```python
from build123d import *

# Parameters (mm, degrees)
SKETCH_1_W      = 100
SKETCH_1_H      = 100
EXTRUDE_1_DEPTH = 3
SKETCH_4_W      = 100
SKETCH_4_H      = 100
EXTRUDE_4_DEPTH = 33
FILLET_3_R      = 8
SKETCH_7_R      = 3.25
EXTRUDE_6_DEPTH = 33


with BuildPart() as part:
    # Эскиз1 → Бобышка-Вытянуть1 (new body)
    with BuildSketch(Plane(origin=(0, 0, 0), x_dir=(1, 0, 0), z_dir=(0, 1, 0))):
        with Locations((50, 50)):
            Rectangle(SKETCH_1_W, SKETCH_1_H)
    extrude(amount=EXTRUDE_1_DEPTH)

    # Эскиз4 → Бобышка-Вытянуть4 (add)
    with BuildSketch(Plane(origin=(0, 3, 0), x_dir=(1, 0, 0), z_dir=(0, 1, 0))):
        with Locations((50, 50)):
            Rectangle(SKETCH_4_W, SKETCH_4_H)
        with BuildLine():
            Line((97, 97), (3, 97))
            Line((3, 97), (3, 64))
            ThreePointArc((3, 64), (2.899494937, 62.585786438), (2.6, 61.2))
            ThreePointArc((2.6, 61.2), (1, 50), (2.6, 38.8))
            ThreePointArc((2.6, 38.8), (2.899494937, 37.414213562), (3, 36))
            Line((3, 36), (3, 3))
            Line((3, 3), (97, 3))
            Line((97, 3), (97, 38.33809621))
            ThreePointArc((97, 38.33809621), (97.143892394, 40.02840472), (97.571428571, 41.670068722))
            ThreePointArc((97.571428571, 41.670068722), (99, 50), (97.571428571, 58.329931278))
            ThreePointArc((97.571428571, 58.329931278), (97.143892394, 59.97159528), (97, 61.66190379))
            Line((97, 61.66190379), (97, 97))
        make_face(mode=Mode.SUBTRACT)
    extrude(amount=EXTRUDE_4_DEPTH)

    # Скругление3
    fillet_3_edges = [part.edges().sort_by_distance(p)[0] for p in [
        (0, 18, -100),
        (100, 18, -100),
        (100, 18, 0),
        (0, 18, 0),
    ]]
    fillet(fillet_3_edges, radius=FILLET_3_R)

    # Эскиз7 → Бобышка-Вытянуть6 (add)
    # profile 1 of 4: a face of its own
    with BuildSketch(Plane(origin=(0, 3, 0), x_dir=(1, 0, 0), z_dir=(0, 1, 0))):
        with BuildLine():
            Line((7, 88.4), (2.4, 88.4))
            Line((2.4, 88.4), (2.4, 97.6))
            Line((2.4, 97.6), (11.6, 97.6))
            Line((11.6, 97.6), (11.6, 93))
            ThreePointArc((11.6, 93), (10.252691193, 89.747308807), (7, 88.4))
        make_face()
        with Locations(Location((7, 93, 0), (0, 0, 270))):
            Circle(SKETCH_7_R, mode=Mode.SUBTRACT)
    # profile 2 of 4: a face of its own
    with BuildSketch(Plane(origin=(0, 3, 0), x_dir=(1, 0, 0), z_dir=(0, 1, 0))):
        with BuildLine():
            Line((93, 88.4), (97.6, 88.4))
            Line((97.6, 88.4), (97.6, 97.6))
            Line((97.6, 97.6), (88.4, 97.6))
            Line((88.4, 97.6), (88.4, 93))
            ThreePointArc((88.4, 93), (89.747308807, 89.747308807), (93, 88.4))
        make_face()
        with Locations(Location((93, 93, 0), (0, 0, 90))):
            Circle(SKETCH_7_R, mode=Mode.SUBTRACT)
    # profile 3 of 4: a face of its own
    with BuildSketch(Plane(origin=(0, 3, 0), x_dir=(1, 0, 0), z_dir=(0, 1, 0))):
        with BuildLine():
            Line((88.4, 7), (88.4, 2.4))
            Line((88.4, 2.4), (97.6, 2.4))
            Line((97.6, 2.4), (97.6, 11.6))
            Line((97.6, 11.6), (93, 11.6))
            ThreePointArc((93, 11.6), (89.747308807, 10.252691193), (88.4, 7))
        make_face()
        with Locations(Location((93, 7, 0), (0, 0, 270))):
            Circle(SKETCH_7_R, mode=Mode.SUBTRACT)
    # profile 4 of 4: a face of its own
    with BuildSketch(Plane(origin=(0, 3, 0), x_dir=(1, 0, 0), z_dir=(0, 1, 0))):
        with BuildLine():
            Line((11.6, 7), (11.6, 2.4))
            Line((11.6, 2.4), (2.4, 2.4))
            Line((2.4, 2.4), (2.4, 11.6))
            Line((2.4, 11.6), (7, 11.6))
            ThreePointArc((7, 11.6), (10.252691193, 10.252691193), (11.6, 7))
        make_face()
        with Locations(Location((7, 7, 0), (0, 0, 90))):
            Circle(SKETCH_7_R, mode=Mode.SUBTRACT)
    extrude(amount=EXTRUDE_6_DEPTH)


solid = part.part
```
Here's how the part is built. I have some questions about the finished solid (model axes, mm). A direction names the side the tool comes from. Give positions to 0.01 mm unless a question says otherwise; leave off trailing zeros. Order: outer loops, then holes, each group sorted by start corner. A loop starts at its lowest first (then second) coordinate and runs counter-clockwise, first axis right, second up. Notation, with made-up numbers: M 22,84.5 L 58,84.5 A38 ccw 58,123.5 Z; hole C 82.25,-25 d10. An arc over 180 degrees is marked long. Use a Markdown table: item, result. Add a question column.
1. Suppose I cut it at A-A (x = 16.5). List the corners of the cut face in (y, z) for me.
2. Suppose I cut it at B-B (z = -44.5). List the corners of the cut face in (x, y) for me, and give its area (3 significant figures).
3. I need wall thicknesses on probe 1 along X at (y, z) = (24.5, -93); probe 2 along Z at (x, y) = (27, 20.5); probe 3 along X at (y, z) = (29, -19.5). Which ranges of each line are inside material? Lowest first, please. Write a range as from..to.
4. Suppose I cut it at C-C (y = 22.5). Give the number of separate pieces and of enclosed holes in the cut face, and give its area (3 significant figures).
5. On a 3-axis mill with a long thin cutter (end or side, diameter ignored), from which of +Z, -Z, +X, -X, +Y, -Y can I reach the whole of each face in a straight line? I mean faces 1 (the cylindrical face through (97.594, 18.252, -2.281)), 2 (the cylindrical face through (89.783, 19.269, -10.288)). Say none if no direction works.
6. For pin 1 Ø3 at (y, z) = (26.5, -5.5) entering from -X; pin 2 Ø5 at (x, z) = (93, -93) entering from +Y; pin 3 Ø2 at (x, y) = (94.5, 19.5) entering from -Z, each with a flat end and sliding along its axis, tell me the tip position at first contact or that it passes through.
7. If we mould it in two halves opening along Z, with no side actions, what happens to faces 3 (the cylindrical face through (2.281, 17.748, -97.594)), 4 (the cylindrical face through (7.143, 19.269, -96.247)), 5 (the flat face through (0, 18, -49)), 6 (the flat face through (3, 19, -24))? For each: +Z half, -Z half, draft (parallel to the pull), parting line (faces both ways), or undercut.
Results list:
| question | item | result |
|---|---|---|
| 1 | outline | M 0,-100 L 36,-100 L 36,-97 L 3,-97 L 3,-3 L 36,-3 L 36,0 L 0,0 Z |
| 2 | outline | M 0,0 L 100,0 L 100,36 L 98.39,36 L 98.39,3 L 1.38,3 L 1.38,36 L 0,36 Z |
| 2 | area | 399 mm² |
| 3 | probe 1 | x = 0.06..3.75, 10.25..11.6, 88.4..89.75, 96.25..99.94 |
| 3 | probe 2 | z = -100..-97, -3..0 |
| 3 | probe 3 | x = 0..3, 97..100 |
| 4 | separate pieces | 1 |
| 4 | enclosed holes | 5 |
| 4 | area | 1,190 mm² |
| 5 | face 1 | +Z, +X, +Y, -Y |
| 5 | face 2 | +Y |
| 6 | pin 1 | stops at x = 0.06 |
| 6 | pin 2 | stops at y = 3 |
| 6 | pin 3 | stops at z = -99.86 |
| 7 | face 3 | -Z half |
| 7 | face 4 | undercut |
| 7 | face 5 | draft |
| 7 | face 6 | undercut |
